Part model, mm, in its own coordinate system. Coordinates: 2 decimals unless noted, no trailing zeros. One line per question, with ' | ' between items. Start each with the question number.
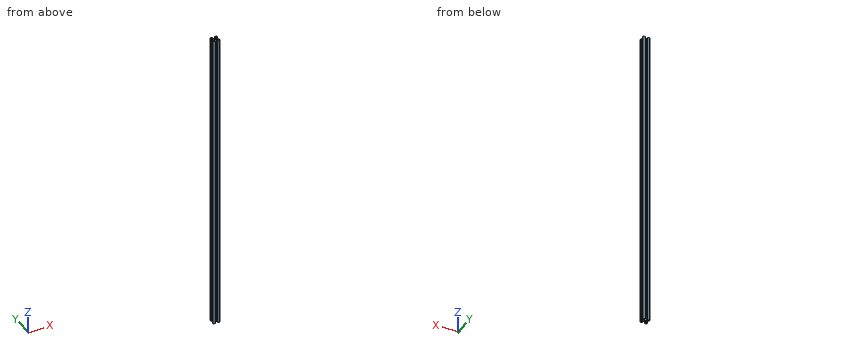
from build123d import *

# Parameters (mm, degrees)
SKETCH1_R      = 3.4
EXTRUDE1_DEPTH = 1400
EXTRUDE2_DEPTH = 1401.160705062


with BuildPart() as part:
    # Sketch1 → Extrude1 (new body)
    with BuildSketch(Plane.XY):
        with BuildLine():
            Line((-5.1, 14.2), (-5.1, 15))
            Line((-5.1, 15), (-12.5, 15))
            ThreePointArc((-12.5, 15), (-14.267766953, 14.267766953), (-15, 12.5))
            Line((-15, 12.5), (-15, 5.1))
            Line((-15, 5.1), (-14.2, 5.1))
            Line((-14.2, 5.1), (-14.2, 4.1))
            Line((-14.2, 4.1), (-13.2, 4.1))
            Line((-13.2, 4.1), (-13.2, 8.25))
            Line((-13.2, 8.25), (-9.522792206, 8.25))
            Line((-9.522792206, 8.25), (-5.7, 4.427207794))
            Line((-5.7, 4.427207794), (-5.7, -4.427207794))
            Line((-5.7, -4.427207794), (-9.522792206, -8.25))
            Line((-9.522792206, -8.25), (-13.2, -8.25))
            Line((-13.2, -8.25), (-13.2, -4.1))
            Line((-13.2, -4.1), (-14.2, -4.1))
            Line((-14.2, -4.1), (-14.2, -5.1))
            Line((-14.2, -5.1), (-15, -5.1))
            Line((-15, -5.1), (-15, -12.5))
            ThreePointArc((-15, -12.5), (-14.267766953, -14.267766953), (-12.5, -15))
            Line((-12.5, -15), (-5.1, -15))
            Line((-5.1, -15), (-5.1, -14.2))
            Line((-5.1, -14.2), (-4.1, -14.2))
            Line((-4.1, -14.2), (-4.1, -13.2))
            Line((-4.1, -13.2), (-8.25, -13.2))
            Line((-8.25, -13.2), (-8.25, -9.522792206))
            Line((-8.25, -9.522792206), (-4.427207794, -5.7))
            Line((-4.427207794, -5.7), (4.427207794, -5.7))
            Line((4.427207794, -5.7), (8.25, -9.522792206))
            Line((8.25, -9.522792206), (8.25, -13.2))
            Line((8.25, -13.2), (4.1, -13.2))
            Line((4.1, -13.2), (4.1, -14.2))
            Line((4.1, -14.2), (5.1, -14.2))
            Line((5.1, -14.2), (5.1, -15))
            Line((5.1, -15), (12.5, -15))
            ThreePointArc((12.5, -15), (14.267766953, -14.267766953), (15, -12.5))
            Line((15, -12.5), (15, -5.1))
            Line((15, -5.1), (14.2, -5.1))
            Line((14.2, -5.1), (14.2, -4.1))
            Line((14.2, -4.1), (13.2, -4.1))
            Line((13.2, -4.1), (13.2, -8.25))
            Line((13.2, -8.25), (9.522792206, -8.25))
            Line((9.522792206, -8.25), (5.7, -4.427207794))
            Line((5.7, -4.427207794), (5.7, 4.427207794))
            Line((5.7, 4.427207794), (9.522792206, 8.25))
            Line((9.522792206, 8.25), (13.2, 8.25))
            Line((13.2, 8.25), (13.2, 4.1))
            Line((13.2, 4.1), (14.2, 4.1))
            Line((14.2, 4.1), (14.2, 5.1))
            Line((14.2, 5.1), (15, 5.1))
            Line((15, 5.1), (15, 12.5))
            ThreePointArc((15, 12.5), (14.267766953, 14.267766953), (12.5, 15))
            Line((12.5, 15), (5.1, 15))
            Line((5.1, 15), (5.1, 14.2))
            Line((5.1, 14.2), (4.1, 14.2))
            Line((4.1, 14.2), (4.1, 13.2))
            Line((4.1, 13.2), (8.25, 13.2))
            Line((8.25, 13.2), (8.25, 9.522792206))
            Line((8.25, 9.522792206), (4.427207794, 5.7))
            Line((4.427207794, 5.7), (-4.427207794, 5.7))
            Line((-4.427207794, 5.7), (-8.25, 9.522792206))
            Line((-8.25, 9.522792206), (-8.25, 13.2))
            Line((-8.25, 13.2), (-4.1, 13.2))
            Line((-4.1, 13.2), (-4.1, 14.2))
            Line((-4.1, 14.2), (-5.1, 14.2))
        make_face()
        Circle(SKETCH1_R, mode=Mode.SUBTRACT)
    extrude(amount=EXTRUDE1_DEPTH)

    # Sketch2 → Extrude2 (cut, through all)
    with BuildSketch(Plane.XY.offset(1400)):
        with BuildLine():
            Line((13.7, 12.7), (13.7, 10.55))
            ThreePointArc((13.7, 10.55), (13.407106781, 9.842893219), (12.7, 9.55))
            Line((12.7, 9.55), (10.55, 9.55))
            ThreePointArc((10.55, 9.55), (9.842893219, 9.842893219), (9.55, 10.55))
            Line((9.55, 10.55), (9.55, 12.7))
            ThreePointArc((9.55, 12.7), (9.842893219, 13.407106781), (10.55, 13.7))
            Line((10.55, 13.7), (12.7, 13.7))
            ThreePointArc((12.7, 13.7), (13.407106781, 13.407106781), (13.7, 12.7))
        make_face()
        with BuildLine():
            Line((-12.7, 13.7), (-10.55, 13.7))
            ThreePointArc((-10.55, 13.7), (-9.842893219, 13.407106781), (-9.55, 12.7))
            Line((-9.55, 12.7), (-9.55, 10.55))
            ThreePointArc((-9.55, 10.55), (-9.842893219, 9.842893219), (-10.55, 9.55))
            Line((-10.55, 9.55), (-12.7, 9.55))
            ThreePointArc((-12.7, 9.55), (-13.407106781, 9.842893219), (-13.7, 10.55))
            Line((-13.7, 10.55), (-13.7, 12.7))
            ThreePointArc((-13.7, 12.7), (-13.407106781, 13.407106781), (-12.7, 13.7))
        make_face()
        with BuildLine():
            Line((12.7, -13.7), (10.55, -13.7))
            ThreePointArc((10.55, -13.7), (9.842893219, -13.407106781), (9.55, -12.7))
            Line((9.55, -12.7), (9.55, -10.55))
            ThreePointArc((9.55, -10.55), (9.842893219, -9.842893219), (10.55, -9.55))
            Line((10.55, -9.55), (12.7, -9.55))
            ThreePointArc((12.7, -9.55), (13.407106781, -9.842893219), (13.7, -10.55))
            Line((13.7, -10.55), (13.7, -12.7))
            ThreePointArc((13.7, -12.7), (13.407106781, -13.407106781), (12.7, -13.7))
        make_face()
        with BuildLine():
            Line((-13.7, -12.7), (-13.7, -10.55))
            ThreePointArc((-13.7, -10.55), (-13.407106781, -9.842893219), (-12.7, -9.55))
            Line((-12.7, -9.55), (-10.55, -9.55))
            ThreePointArc((-10.55, -9.55), (-9.842893219, -9.842893219), (-9.55, -10.55))
            Line((-9.55, -10.55), (-9.55, -12.7))
            ThreePointArc((-9.55, -12.7), (-9.842893219, -13.407106781), (-10.55, -13.7))
            Line((-10.55, -13.7), (-12.7, -13.7))
            ThreePointArc((-12.7, -13.7), (-13.407106781, -13.407106781), (-13.7, -12.7))
        make_face()
    extrude(amount=-EXTRUDE2_DEPTH, mode=Mode.SUBTRACT)


solid = part.part
1) Band-saw the part on A-A on z = 986.5. Count the separate pieces of the cut face and the enclosed holes in it, then the cut area to 3 significant figures.
2) Wall check: line 1 along X through (y, z) = (-11, 1167.5); line 2 along Y through (x, z) = (13, 94). Give the ranges that are in metal, low to high. Write a range as [from, to].
3) Pin check, flat tips, straight feed: pin 1 Ø4 at (y, z) = (-4, 1230) entering from +X; pin 2 Ø0.8 at (x, z) = (-13.5, 372.5) entering from +Y; pin 3 Ø0.8 at (x, z) = (-13.5, 467.5) entering from -Y; pin 4 Ø3 at (x, z) = (3.5, 812) entering from +Y. Stop position of each tip, or through.
Values found:
1) separate pieces: 1 | enclosed holes: 5 | area: 291 mm²
2) line 1: [-15, -13.7], [-9.55, -8.25], [8.25, 9.55], [13.7, 15] | line 2: [-14.95, -13.65], [-9.6, -8.25], [8.25, 9.6], [13.65, 14.95]
3) pin 1: x = 15 | pin 2: y = 14.93 | pin 3: y = -14.93 | pin 4: y = 14.2
